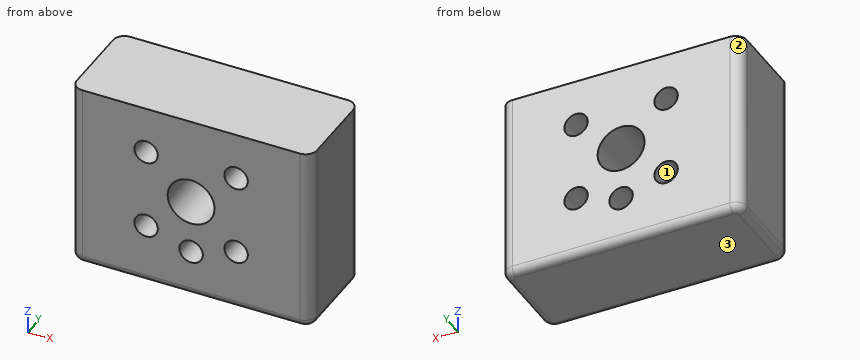
```python
from build123d import *

# Parameters (mm, degrees)
F1_DEPTH = 200
F3_D     = 25
F4_R     = 8
F5_D     = 50


with BuildPart() as f1:
    # F0 (on Top) → F1 (new body)
    with BuildSketch(Plane.XY):
        with BuildLine():
            Line((116, 50), (-116, 50))
            ThreePointArc((-116, 50), (-124.485281, 46.485281), (-128, 38))
            Line((-128, 38), (-128, -38))
            ThreePointArc((-128, -38), (-124.485281, -46.485281), (-116, -50))
            Line((-116, -50), (116, -50))
            ThreePointArc((116, -50), (124.485281, -46.485281), (128, -38))
            Line((128, -38), (128, 38))
            ThreePointArc((128, 38), (124.485281, 46.485281), (116, 50))
        make_face()
    extrude(amount=-F1_DEPTH)

    # F3 (through all)
    with Locations(Plane.XZ.offset(50)):
        with Locations((-48, -50), (48, -50), (48, -135), (0, -150), (-48, -135)):
            Hole(F3_D / 2)

    # F4
    f4_edges = [f1.edges().sort_by_distance(p)[0] for p in [
        (128, 0, -200),
    ]]
    fillet(f4_edges, radius=F4_R)

    # F5 (through all)
    with Locations(Plane.XZ.offset(50)):
        with Locations((0, -92.5)):
            Hole(F5_D / 2)


solid = f1.part
```
Read the model definition and answer for the solid it produces. Units are mm, in the model's axes. Face numbers are marked on the shaded views. Coordinates: 2 decimals unless noted, no trailing zeros. Loops run counter-clockwise (first coordinate to the right, second up) from the corner with the lowest first, then second, coordinate; pieces in that order, holes last. Notation, with made-up numbers: (42, -14.75) - (91, -14.75) arc R10 cw to (91, 4.25) - close; hole circle Ø11 at (-14, 70). An arc over 180 degrees is marked (long way). Answer in a Markdown table with one row per item.
1. Find section A-A, the plane x = 0. Write down the section's boundary in (y, z), then the cut area to 3 significant figures.
Conclusion:
| item | result |
|---|---|
| outline | (-50, -192) arc R8 ccw to (-42, -200) - (42, -200) arc R8 ccw to (50, -192) - (50, -162.5) - (-50, -162.5) - close; (-50, -137.5) - (50, -137.5) - (50, -117.5) - (-50, -117.5) - close; (-50, -67.5) - (50, -67.5) - (50, 0) - (-50, 0) - close |
| area | 12,500 mm² |
2. Find section D-D, the plane x = 48. Write down the section's boundary in (y, z).
Conclusion:
| item | result |
|---|---|
| outline | (-50, -192) arc R8 ccw to (-42, -200) - (42, -200) arc R8 ccw to (50, -192) - (50, -147.5) - (-50, -147.5) - close; (-50, -122.5) - (50, -122.5) - (50, -62.5) - (-50, -62.5) - close; (-50, -37.5) - (50, -37.5) - (50, 0) - (-50, 0) - close |
3. Determine the mould class of the marked faces 1, 2 and 3 for opening direction X: +X half, -X half, draft (parallel to the pull), parting line (faces both ways), or undercut.
Conclusion:
| item | result |
|---|---|
| face 1 | undercut |
| face 2 | -X half |
| face 3 | draft |
4. Find section C-C, the plane y = 15. Write down the section's boundary in (x, z).
Conclusion:
| item | result |
|---|---|
| outline | (-128, -192) arc R8 ccw to (-120, -200) - (120, -200) arc R8 ccw to (128, -192) - (128, 0) - (-128, 0) - close; hole circle Ø25 at (-48, -135); hole circle Ø25 at (-48, -50); hole circle Ø50 at (0, -92.5); hole circle Ø25 at (0, -150); hole circle Ø25 at (48, -135); hole circle Ø25 at (48, -50) |
5. Straight lines are drawn through the part: line 1 (Z direction, x = -48, y = 12); line 2 (Z direction, x = 0, y = 13); line 3 (X direction, y = -6, z = -126). For each, find the intervals that lie inside material, in ascending order.
Conclusion:
| item | result |
|---|---|
| line 1 | z = -200 to -147.5, -122.5 to -62.5, -37.5 to 0 |
| line 2 | z = -200 to -162.5, -137.5 to -117.5, -67.5 to 0 |
| line 3 | x = -128 to -56.67, -39.33 to 39.33, 56.67 to 128 |
6. Find section B-B, the plane z = -92.5. Write down the section's boundary in (x, y), then the cut area to 3 significant figures.
Conclusion:
| item | result |
|---|---|
| outline | (-128, -38) arc R12 ccw to (-116, -50) - (-25, -50) - (-25, 50) - (-116, 50) arc R12 ccw to (-128, 38) - close; (25, -50) - (116, -50) arc R12 ccw to (128, -38) - (128, 38) arc R12 ccw to (116, 50) - (25, 50) - close |
| area | 20,500 mm² |
7. Given pin 1 (22.5 mm diameter, centred on x = 48, z = -135, fed in from +Y), flat-ended and moving along its own axis, determine where the tip first touches the part or whether it passes through.
Conclusion:
| item | result |
|---|---|
| pin 1 | passes through |
